```python
from build123d import *

# Parameters (mm, degrees)
EXTRUDE_1_DEPTH     = 6
SKETCH_2_R          = 9
EXTRUDE_2_DEPTH     = 6
SKETCH_3_R          = 6
SKETCH_3_R_2        = 3
CUT_EXTRUDE_1_DEPTH = 6
FILLET_1_R          = 10
CUT_EXTRUDE_2_DEPTH = 6


with BuildPart() as part:
    # 草图1 → 凸台-拉伸1 (new body)
    with BuildSketch(Plane.XY):
        with BuildLine():
            Line((-6, -52), (-6, 52))
            ThreePointArc((-6, 52), (0, 58), (6, 52))
            Line((6, 52), (6, -52))
            ThreePointArc((6, -52), (0, -58), (-6, -52))
        make_face()
    extrude(amount=EXTRUDE_1_DEPTH)

    # 草图2 → 凸台-拉伸2 (add)
    with BuildSketch(Plane(origin=(0, 0, 0), x_dir=(-1, 0, 0), z_dir=(0, 0, -1))):
        with Locations((0, -52)):
            Circle(SKETCH_2_R)
    extrude(amount=-EXTRUDE_2_DEPTH)

    # 草图3 → 切除-拉伸1 (cut)
    with BuildSketch(Plane(origin=(0, 0, 0), x_dir=(-1, 0, 0), z_dir=(0, 0, -1))):
        with Locations((0, -52)):
            Circle(SKETCH_3_R)
        with Locations((0, 52)):
            Circle(SKETCH_3_R_2)
    extrude(amount=-CUT_EXTRUDE_1_DEPTH, mode=Mode.SUBTRACT)

    # 圆角1
    fillet_1_edges = [part.edges().sort_by_distance(p)[0] for p in [
        (6, -45.291796068, 3),
        (-6, -45.291796068, 3),
    ]]
    fillet(fillet_1_edges, radius=FILLET_1_R)

    # 草图4 → 切除-拉伸2 (cut)
    with BuildSketch(Plane.XY.offset(6)):
        with BuildLine():
            Line((-2, -39), (-2, 39))
            ThreePointArc((-2, 39), (0, 41), (2, 39))
            Line((2, 39), (2, -39))
            ThreePointArc((2, -39), (0, -41), (-2, -39))
        make_face()
    extrude(amount=-CUT_EXTRUDE_2_DEPTH, mode=Mode.SUBTRACT)


solid = part.part
```
Check sheet for the modelled part. Datum: model origin and axes. Units: mm. A direction names the side the tool comes from. Round coordinates to 2 decimals unless told otherwise and drop trailing zeros. Order: outer loops, then holes, each group sorted by start corner. A loop starts at its lowest first (then second) coordinate and runs counter-clockwise, first axis right, second up.
1) Section check C-C (y = 4.5). Record the boundary of the cut face in (x, z).
2) Section check D-D (x = 4.5). Record the boundary of the cut face in (y, z), and give its area (3 significant figures).
3) Scan lines: line 1 (Y direction, x = 0, z = 3.3); line 2 (X direction, y = 6.5, z = 0.65); line 3 (Y direction, x = -1.75, z = 1.7). Record each from-to range of solid material in increasing order.
4) Tool access check on faces 4 (the flat face through (-4, -1, 6)), 5 (the cylindrical face through (0, 41, 3)), 6 (the flat face through (-6, 4, 3)), 7 (the flat face through (6, 6, 3)). Record the directions out of +Z, -Z, +X, -X, +Y, -Y that give a thin tool (end or side, any length) a straight path to the whole face; none if there is none.
5) Mould release check, pull along Y, two halves, no side actions. Record for faces 1 (the cylindrical face through (6.414, -44.601, 2.958)), 2 (the cylindrical face through (0, -61, 3)), 3 (the flat face through (2, 1, 3)): +Y half, -Y half, draft (parallel to the pull), parting line (faces both ways), or undercut.
6) Go/stop test with flat-tipped pins: pin 1 Ø1.5 at (x, z) = (3, 1.5) entering from +Y; pin 2 Ø3 at (y, z) = (-2, 3) entering from -X; pin 3 Ø1.5 at (x, z) = (6.5, 0.5) entering from -Y. Record where each tip stops, or that it passes through.
7) Section check B-B (z = 4.9). Record the boundary of the cut face in (x, y).
8) Section check A-A (x = 0). Record the boundary of the cut face in (y, z).
Result:
1. outline: (-6, 0) - (-2, 0) - (-2, 6) - (-6, 6) - close; (2, 0) - (6, 0) - (6, 6) - (2, 6) - close
2. outline: (-59.79, 0) - (-55.97, 0) - (-55.97, 6) - (-59.79, 6) - close; (-48.03, 0) - (55.97, 0) - (55.97, 6) - (-48.03, 6) - close
2. area: 647 mm2
3. line 1: y = -61 to -58, -46 to -41, 41 to 49, 55 to 58
3. line 2: x = -6 to -2, 2 to 6
3. line 3: y = -60.83 to -57.74, -46.26 to -39.97, 39.97 to 49.56, 54.44 to 57.74
4. face 4: +Z, +X, -X, +Y, -Y
4. face 5: +Z, -Z
4. face 6: +Z, -Z, -X, +Y
4. face 7: +Z, -Z, +X, +Y
5. face 1: +Y half
5. face 2: parting line
5. face 3: undercut
6. pin 1: stops at y = 57.56
6. pin 2: stops at x = -6
6. pin 3: stops at y = -58.92
7. outline: (-7.58, -47.15) arc R9 ccw (long way) to (7.58, -47.15) arc R10 cw to (6, -41.75) - (6, 52) arc R6 ccw to (-6, 52) - (-6, -41.75) arc R10 cw to start; hole circle Ø12 at (0, -52); hole circle Ø6 at (0, 52); hole (-2, -39) arc R2 ccw to (2, -39) - (2, 39) arc R2 ccw to (-2, 39) - close
8. outline: (-61, 0) - (-58, 0) - (-58, 6) - (-61, 6) - close; (-46, 0) - (-41, 0) - (-41, 6) - (-46, 6) - close; (41, 0) - (49, 0) - (49, 6) - (41, 6) - close; (55, 0) - (58, 0) - (58, 6) - (55, 6) - close
